```python
from build123d import *

# Parameters (mm, degrees)
ESBO_O2_OUTSIDE_W          = 45.75
ESBO_O2_OUTSIDE_H          = 45.75
ESBO_O2_OUTSIDE_W_2        = 30
ESBO_O2_OUTSIDE_H_2        = 15
CORTE_EXTRUS_O1_DEPTH      = 28.05
CORTE_EXTRUS_O1_DEPTH_BACK = 28.05
CORTE_EXTRUS_O2_DEPTH      = 16


with BuildPart() as part:
    # Esboço1 one side → Revolução1 (revolve)
    with BuildSketch(Plane.XY):
        with BuildLine():
            ThreePointArc((4, 26.506832295), (2.018355219, 26.913587797), (0, 27.05))
            Line((0, 27.05), (0, -27.05))
            ThreePointArc((0, -27.05), (2.018355219, -26.913587797), (4, -26.506832295))
            Line((4, -26.506832295), (15, -12.05))
            Line((15, -12.05), (9.95, -12.05))
            Line((9.95, -12.05), (9.95, 12.05))
            Line((9.95, 12.05), (15, 12.05))
            Line((15, 12.05), (4, 26.506832295))
        make_face()
    revolve(axis=Axis((0, -27.05, 0), (0, 1, 0)))

    # Esboço2 outside → Corte-extrusão1 (cut, two sides)
    with BuildSketch(Plane(origin=(0, 0, 0), x_dir=(1, 0, 0), z_dir=(0, 1, 0))) as corte_extrus_o1_sk:
        Rectangle(ESBO_O2_OUTSIDE_W, ESBO_O2_OUTSIDE_H)
        Rectangle(ESBO_O2_OUTSIDE_W_2, ESBO_O2_OUTSIDE_H_2, mode=Mode.SUBTRACT)
    extrude(amount=CORTE_EXTRUS_O1_DEPTH, mode=Mode.SUBTRACT)
    extrude(corte_extrus_o1_sk.sketch, amount=-CORTE_EXTRUS_O1_DEPTH_BACK, mode=Mode.SUBTRACT)

    # Esboço3 → Corte-extrusão2 (cut, through all)
    with BuildSketch(Plane(origin=(0, 0, -7.5), x_dir=(-1, 0, 0), z_dir=(0, 0, -1))):
        with BuildLine():
            Line((6, 27.05), (6, 12.55))
            ThreePointArc((6, 12.55), (0, 6.55), (-6, 12.55))
            Line((-6, 12.55), (-6, 27.05))
            ThreePointArc((-6, 27.05), (0, 33.05), (6, 27.05))
        make_face()
        with BuildLine():
            Line((-5, -27.05), (-5, -12.55))
            ThreePointArc((-5, -12.55), (0, -7.55), (5, -12.55))
            Line((5, -12.55), (5, -27.05))
            ThreePointArc((5, -27.05), (0, -32.05), (-5, -27.05))
        make_face()
    extrude(amount=-CORTE_EXTRUS_O2_DEPTH, mode=Mode.SUBTRACT)


solid = part.part
```
Here's how the part is built. I have some questions about the finished solid (model axes, mm). A direction names the side the tool comes from. Round coordinates to 2 decimals unless told otherwise and drop trailing zeros. Loops run counter-clockwise (first coordinate to the right, second up) from the corner with the lowest first, then second, coordinate; pieces in that order, holes last. Notation, with made-up numbers: (70, -18) -> (107, -18) arc R6 ccw to (107, -14) -> close; hole circle Ø7 at (-35.75, 36). An arc over 180 degrees is marked (long way). Answer as CSV lines item,"result". Start each with the question number.
1. For faces 5 (the face through (5, -18, 0)), 6 (the face through (9.95, 0.17, 0.12)), 7 (the face through (-6, 17, 0)), 8 (the face through (-12, -12.05, 0)), which set-ups out of +Z, -Z, +X, -X, +Y, -Y let a thin tool reach every point of the face, with its end or its side?
2. Imagine slicing it at B-B on y = -16. Write out the boundary of the cut face in (x, z), plus the area to 3 significant figures.
3. Imagine slicing it at A-A on y = -8.5. Write out the boundary of the cut face in (x, z).
4. If we mould it in two halves opening along X, with no side actions, what happens to faces 1 (the face through (10.07, -18.53, 0.14)), 2 (the face through (0.11, -7.55, -0.11)), 3 (the face through (6, 17, 0)), 4 (the face through (-10.402, 18.091, -0.131))? For each: pulls with the +X half, pulls with the -X half, needs draft (parallel to the pull), parting line crosses it, or undercut.
5. Imagine slicing it at C-C on x = 0. Write out the boundary of the cut face in (y, z).
6. Imagine slicing it at D-D on y = 5. Write out the boundary of the cut face in (x, z), plus the area to 3 significant figures.
7. I'm going to push flat-ended pins straight in: P1, Ø6, axis at x = -2.5, z = 0.5, coming from the +Y side; P2, Ø6.5, axis at y = -18, z = 0.5, coming from the -X side; P3, Ø9, axis at y = 19.5, z = 2, coming from the +X side. Where does each tip first touch, or does it pass through?
Solution:
1,face 5,"+Z, -Z, -Y"
1,face 6,"+X"
1,face 7,"+Z, -Z, +Y"
1,face 8,"-X"
2,outline,"(-9.36, -7.5) -> (-5, -7.5) -> (-5, 7.5) -> (-9.36, 7.5) arc R11.99 ccw to start; (5, -7.5) -> (9.36, -7.5) arc R11.99 ccw to (9.36, 7.5) -> (5, 7.5) -> close"
2,area,"185 mm²"
3,outline,"(-6.54, -7.5) -> (-2.93, -7.5) -> (-2.93, 7.5) -> (-6.54, 7.5) arc R9.95 ccw to start; (2.93, -7.5) -> (6.54, -7.5) arc R9.95 ccw to (6.54, 7.5) -> (2.93, 7.5) -> close"
4,face 1,"pulls with the +X half"
4,face 2,"undercut"
4,face 3,"undercut"
4,face 4,"pulls with the -X half"
5,outline,"(-7.55, -7.5) -> (6.55, -7.5) -> (6.55, 7.5) -> (-7.55, 7.5) -> close"
6,outline,"(-6.54, -7.5) -> (6.54, -7.5) arc R9.95 ccw to (6.54, 7.5) -> (-6.54, 7.5) arc R9.95 ccw to start"
6,area,"267 mm²"
7,P1,"y = 10.15"
7,P2,"x = -12.94"
7,P3,"x = 12.65"
